Geometry check sheet. Reference: drawing and pictorial views, mm from the part's lowest x, y, z. Give positions to 0.01 mm unless a question says otherwise; leave off trailing zeros. Loops run counter-clockwise (first coordinate to the right, second up) from the corner with the lowest first, then second, coordinate; pieces in that order, holes last. Notation, with made-up numbers: M 55.25,47.5 L 103.25,47.5 A19 ccw 103.25,56.5 Z; hole C 54.5,59 d7. An arc over 180 degrees is marked long. One line per question, with ' | ' between items. Start each with the question number.
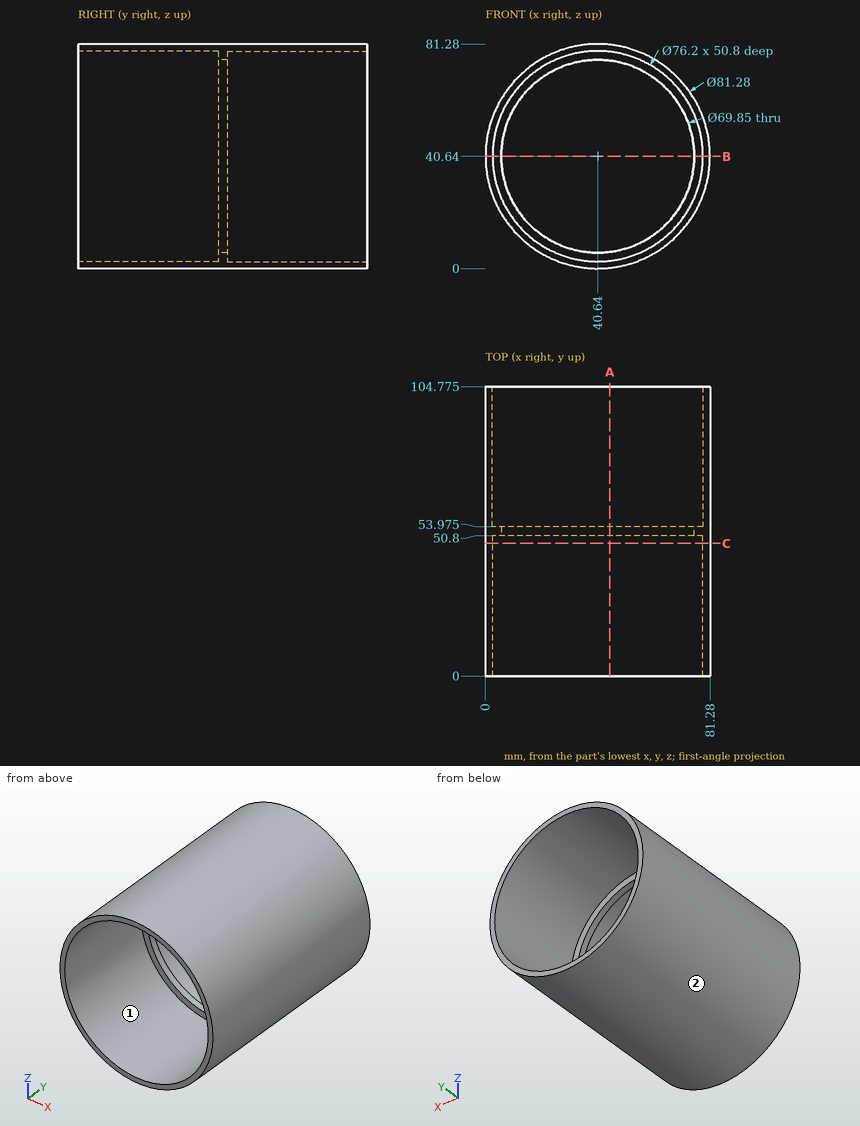
Q1. Cross-section at C-C (y = 48). Record the cut outline in (x, z).
Q2. Depth check by flat-ended pin: P1, Ø2, axis at x = 50, y = 74.5, coming from the -Z side; P2, Ø4, axis at y = 28.5, z = 62, coming from the -X side; P3, Ø8, axis at y = 78.5, z = 62.5, coming from the -X side. Enter the tip coordinate at first touch or a pass-through.
Q3. Cross-section at A-A (x = 45). Record the cut outline in (y, z) (3 decimals).
Q4. Material ranges on probe 1 along Z at (x, y) = (40.64, 53) (3 decimals); probe 2 along Z at (x, y) = (40.64, 78); probe 3 along X at (y, z) = (10, 44), recorded low to high. Write a range as from..to.
Q5. Draft check along Z on the marked faces 1 and 2. Enter one of: released by +Z, released by -Z, zero draft, split by the parting line, or undercut.
Q6. Cross-section at B-B (z = 40.64). Record the cut outline in (x, y) (3 decimals).
Solved:
1) outline: C 40.64,40.64 d81.28; hole C 40.64,40.64 d76.2
2) P1: stops at z = 0.87 | P2: stops at x = 4.91 | P3: stops at x = 4.13
3) outline: M 0,0.235 L 104.775,0.235 L 104.775,2.79 L 53.975,2.79 L 53.975,5.988 L 50.8,5.988 L 50.8,2.79 L 0,2.79 Z; M 0,78.49 L 50.8,78.49 L 50.8,75.292 L 53.975,75.292 L 53.975,78.49 L 104.775,78.49 L 104.775,81.045 L 0,81.045 Z
4) probe 1: z = 0..5.715, 75.565..81.28 | probe 2: z = 0..2.54, 78.74..81.28 | probe 3: x = 0.14..2.69, 78.59..81.14
5) face 1: undercut | face 2: split by the parting line
6) outline: M 0,0 L 2.54,0 L 2.54,50.8 L 5.715,50.8 L 5.715,53.975 L 2.54,53.975 L 2.54,104.775 L 0,104.775 Z; M 75.565,50.8 L 78.74,50.8 L 78.74,0 L 81.28,0 L 81.28,104.775 L 78.74,104.775 L 78.74,53.975 L 75.565,53.975 Z
